Autodesk Inventor part; units mm, degrees
ref_plane "YZ Plane" through (0, 0, 0) normal (1, 0, 0) x (0, 1, 0)
ref_plane "XZ Plane" through (0, 0, 0) normal (0, 1, 0) x (-1, 0, 0)
ref_plane "XY Plane" through (0, 0, 0) normal (0, 0, 1) x (1, 0, 0)
sketch "Sketch1" plane through (0, 0, 0) normal (0, 1, 0) x (-1, 0, 0)
  line L0 (6.35, 0) -> (1365.25, 0)
  line L1 (1371.6, -6.35) -> (1371.6, -1365.25)
  line L2 (1365.25, -1371.6) -> (6.35, -1371.6)
  line L3 (0, -1365.25) -> (0, -6.35)
  line L4 (1346.2, -1346.2) -> (1346.2, -25.4)
  line L5 (1346.2, -25.4) -> (25.4, -25.4)
  line L6 (25.4, -25.4) -> (25.4, -1346.2)
  line L7 (25.4, -1346.2) -> (1346.2, -1346.2)
  line L8 (1320.8, -50.8) -> (1320.8, -1320.8)
  line L9 (1320.8, -1320.8) -> (50.8, -1320.8)
  line L10 (50.8, -1320.8) -> (50.8, -50.8)
  line L11 (50.8, -50.8) -> (1320.8, -50.8)
  line L12 (1320.8, -50.8) -> (1346.2, -25.4)
  line L13 (1320.8, -1320.8) -> (1346.2, -1346.2)
  line L14 (50.8, -1320.8) -> (25.4, -1346.2)
  line L15 (50.8, -50.8) -> (25.4, -25.4)
  line L16 (1219.2, -482.6) -> (1016, -482.6)
  line L17 (1016, -482.6) -> (1016, -889)
  line L18 (1016, -889) -> (1219.2, -889)
  line L19 (1219.2, -889) -> (1219.2, -482.6)
  line L20 (355.6, -482.6) -> (152.4, -482.6)
  line L21 (152.4, -482.6) -> (152.4, -889)
  line L22 (152.4, -889) -> (355.6, -889)
  line L23 (355.6, -889) -> (355.6, -482.6)
  line L24 (889, -1016) -> (482.6, -1016)
  line L25 (482.6, -1016) -> (482.6, -1219.2)
  line L26 (482.6, -1219.2) -> (889, -1219.2)
  line L27 (889, -1219.2) -> (889, -1016)
  line L28 (889, -152.4) -> (482.6, -152.4)
  line L29 (482.6, -152.4) -> (482.6, -355.6)
  line L30 (482.6, -355.6) -> (889, -355.6)
  line L31 (889, -355.6) -> (889, -152.4)
  circle A0 centre (685.8, -685.8) radius 254
  line L32 (889, -127) -> (482.6, -127)
  line L33 (457.2, -127) -> (457.2, -381)
  line L34 (457.2, -381) -> (914.4, -381)
  line L35 (914.4, -381) -> (914.4, -127)
  line L36 (1244.6, -457.2) -> (990.6, -457.2)
  line L37 (990.6, -457.2) -> (990.6, -914.4)
  line L38 (990.6, -914.4) -> (1244.6, -914.4)
  line L39 (1244.6, -889) -> (1244.6, -482.6)
  line L40 (914.4, -990.6) -> (457.2, -990.6)
  line L41 (457.2, -990.6) -> (457.2, -1244.6)
  line L42 (482.6, -1244.6) -> (889, -1244.6)
  line L43 (914.4, -1244.6) -> (914.4, -990.6)
  line L44 (381, -457.2) -> (127, -457.2)
  line L45 (127, -482.6) -> (127, -889)
  line L46 (127, -914.4) -> (381, -914.4)
  line L47 (381, -914.4) -> (381, -457.2)
  line L48 (152.4, -482.6) -> (50.8, -482.6)
  line L49 (127, -457.2) -> (50.8, -457.2)
  line L50 (152.4, -889) -> (50.8, -889)
  line L51 (127, -914.4) -> (50.8, -914.4)
  line L52 (355.6, -889) -> (381, -889)
  line L53 (355.6, -482.6) -> (381, -482.6)
  line L54 (457.2, -1244.6) -> (457.2, -1320.8)
  line L55 (482.6, -1219.2) -> (482.6, -1320.8)
  line L56 (889, -1219.2) -> (889, -1320.8)
  line L57 (914.4, -1244.6) -> (914.4, -1320.8)
  line L58 (1244.6, -914.4) -> (1320.8, -914.4)
  line L59 (1219.2, -889) -> (1320.8, -889)
  line L60 (1219.2, -482.6) -> (1320.8, -482.6)
  line L61 (1244.6, -457.2) -> (1320.8, -457.2)
  line L62 (889, -152.4) -> (889, -50.8)
  line L63 (914.4, -127) -> (914.4, -50.8)
  line L64 (482.6, -152.4) -> (482.6, -50.8)
  line L65 (457.2, -127) -> (457.2, -50.8)
  line L66 (889, -1016) -> (889, -990.6)
  line L67 (482.6, -1016) -> (482.6, -990.6)
  line L68 (1016, -889) -> (990.6, -889)
  line L69 (1016, -482.6) -> (990.6, -482.6)
  line L70 (889, -355.6) -> (889, -381)
  line L71 (482.6, -355.6) -> (482.6, -381)
  line L72 (914.4, -381) -> (990.6, -457.2)
  line L73 (990.6, -482.6) -> (889, -381)
  line L74 (990.6, -914.4) -> (914.4, -990.6)
  line L75 (889, -990.6) -> (990.6, -889)
  line L76 (381, -914.4) -> (457.2, -990.6)
  line L77 (482.6, -990.6) -> (381, -889)
  line L78 (457.2, -381) -> (381, -457.2)
  line L79 (482.6, -381) -> (381, -482.6)
  line L80 (1257.3, -50.8) -> (1320.8, -114.3)
  line L81 (1320.8, -1257.3) -> (1257.3, -1320.8)
  line L82 (50.8, -1257.3) -> (114.3, -1320.8)
  line L83 (50.8, -114.3) -> (114.3, -50.8)
  line L84 (68.7605, -132.2605) -> (132.2605, -68.7605)
  line L85 (68.7605, -1239.3395) -> (132.2605, -1302.8395)
  line L86 (1302.8395, -1239.3395) -> (1239.3395, -1302.8395)
  line L87 (1239.3395, -68.7605) -> (1302.8395, -132.2605)
  line L88 (1302.8395, -132.2605) -> (1320.8, -150.221)
  line L89 (1239.3395, -68.7605) -> (1221.379, -50.8)
  line L90 (1302.8395, -1239.3395) -> (1320.8, -1221.379)
  line L91 (1239.3395, -1302.8395) -> (1221.379, -1320.8)
  line L92 (132.2605, -1302.8395) -> (150.221, -1320.8)
  line L93 (68.7605, -1239.3395) -> (50.8, -1221.379)
  line L94 (132.2605, -68.7605) -> (150.221, -50.8)
  line L95 (68.7605, -132.2605) -> (50.8, -150.221)
  line L96 (1365.25, 0) -> (1371.6, -6.35)
  line L97 (1371.6, -1365.25) -> (1365.25, -1371.6)
  line L98 (6.35, -1371.6) -> (0, -1365.25)
  line L99 (6.35, 0) -> (0, -6.35)
  point P0 (0, 0)
  point P1 (1371.6, -1371.6)
  point P2 (1371.6, 0)
  point P3 (0, -1371.6)
  dimension "d0" = 1371.6
  dimension "d1" = 1371.6
  dimension "d2" = 25.4
  dimension "d3" = 25.4
  dimension "d4" = 203.2
  dimension "d5" = 406.4
  dimension "d6" = 203.2
  dimension "d7" = 406.4
  dimension "d8" = 406.4
  dimension "d9" = 203.2
  dimension "d10" = 406.4
  dimension "d11" = 203.2
  dimension "d12" = 101.6
  dimension "d13" = 101.6
  dimension "d14" = 101.6
  dimension "d15" = 101.6
  dimension "d16" = 431.8
  dimension "d17" = 431.8
  dimension "d18" = 431.8
  dimension "d19" = 431.8
  dimension "d20" = 508
  dimension "d21" = 25.4
  dimension "d22" = 25.4
  dimension "d23" = 25.4
  dimension "d24" = 25.4
  dimension "d25" = 45
  dimension "d26" = 63.5
  dimension "d27" = 45
  dimension "d28" = 45
  dimension "d29" = 45
  dimension "d30" = 25.4
  dimension "d31" = 25.4
  dimension "d32" = 25.4
  dimension "d33" = 25.4
  dimension "d34" = 6.35
  dimension "d35" = 6.35
  dimension "d36" = 6.35
  dimension "d37" = 6.35
  dimension "d38" = 6.35
  dimension "d39" = 6.35
  dimension "d40" = 6.35
  dimension "d41" = 6.35
extrude "Extrusion1" add sketch "Sketch1" along normal blind 5.08 contours L0 L96 L1 L97 L2 L98 L3 L99 | L13 L8 L12 L4 | L7 L14 L9 L13 | L12 L11 L15 L5 | L6 L15 L10 L14 | L9 L81 L8 | L8 L80 L11 | L10 L82 L9 | L81 L9 L91 L86 L90 L8 | L11 L83 L10 | L8 L88 L87 L89 L11 L80 | L82 L10 L93 L85 L92 L9 | L90 L86 L91 L9 L57 L43 L74 L38 L58 L8 | L83 L11 L94 L84 L95 L10 | L8 L61 L36 L72 L35 L63 L11 L89 L87 L88 | L92 L85 L93 L10 L51 L46 L76 L41 L54 L9 | L58 L38 L37 L68 L18 L59 L8 | L9 L56 L27 L66 L40 L43 L57 | L95 L84 L94 L11 L65 L33 L78 L44 L49 L10 | L8 L60 L16 L69 L37 L36 L61 | L63 L35 L34 L70 L31 L62 L11 | L54 L41 L40 L67 L25 L55 L9 | L10 L50 L22 L52 L47 L46 L51 | L59 L39 L60 L8 | L9 L55 L42 L56 | L49 L44 L47 L53 L20 L48 L10 | L11 L64 L29 L71 L34 L33 L65 | L62 L32 L64 L11 | L10 L48 L45 L50 | L74 L40 L75 L37 | L37 L73 L34 L72 | L76 L47 L77 L40 | L75 L40 L77 L47 L79 L34 L73 L37 | L78 L34 L79 L47
chamfer "Chamfer1" distance 1.524 angle 45 8 edges at (-1371.6, 5.08, -685.8) (-1371.6, 0, -685.8) (-685.8, 5.08, 0) (-685.8, 0, 0) (-685.8, 5.08, -1371.6) (-685.8, 0, -1371.6) (0, 5.08, -685.8) (0, 0, -685.8)
properties part number "Glass top X1" material "Glass"
Verification items for the finished model (mm, model axes). Round coordinates to 2 decimals unless told otherwise and drop trailing zeros. Order: outer loops, then holes, each group sorted by start corner. A loop starts at its lowest first (then second) coordinate and runs counter-clockwise, first axis right, second up. Notation, with made-up numbers: (1.5, -10.5) -> (44.5, -10.5) arc R21 cw to (44.5, 16.5) -> close; hole circle Ø5 at (-14.5, 59.25). An arc over 180 degrees is marked (long way). Put each result on its own line as item: value. Start each with the question number.
(1) Depth check by flat-ended pin: pin 1 Ø1 at (y, z) = (1, -867) entering from -X. Enter the tip coordinate at first touch or a pass-through.
(2) Material ranges on line 1 along Z through (x, y) = (-685.8, 2); line 2 along Z through (x, y) = (-685.8, 1.15); line 3 along X through (y, z) = (2.4, -1139), recorded low to high.
(3) Section check D-D (y = 2.45). Enter the section's corners in (x, z).
(4) Section check B-B (z = -685.8). Enter the section's corners in (x, y).
(5) Section check C-C (x = -685.8). Enter the section's corners in (y, z).
(6) Section check A-A (x = -1200). Enter the section's corners in (y, z).
Completed:
1. pin 1: stops at x = -1371.58
2. line 1: z = -1371.6 to -1244.6, -990.6 to -939.8, -431.8 to -381, -127 to 0
2. line 2: z = -1371.23 to -1244.6, -990.6 to -939.8, -431.8 to -381, -127 to -0.37
2. line 3: x = -1371.6 to -889, -482.6 to 0
3. outline: (-1371.6, -1365.25) -> (-1365.25, -1371.6) -> (-6.35, -1371.6) -> (0, -1365.25) -> (0, -6.35) -> (-6.35, 0) -> (-1365.25, 0) -> (-1371.6, -6.35) -> close; hole (-1244.6, -889) -> (-990.6, -889) -> (-990.6, -482.6) -> (-1244.6, -482.6) -> close; hole circle Ø508 at (-685.8, -685.8); hole (-889, -1244.6) -> (-482.6, -1244.6) -> (-482.6, -990.6) -> (-889, -990.6) -> close; hole (-889, -381) -> (-482.6, -381) -> (-482.6, -127) -> (-889, -127) -> close; hole (-381, -889) -> (-127, -889) -> (-127, -482.6) -> (-381, -482.6) -> close
4. outline: (-1371.6, 1.52) -> (-1370.08, 0) -> (-1244.6, 0) -> (-1244.6, 5.08) -> (-1370.08, 5.08) -> (-1371.6, 3.56) -> close; (-990.6, 0) -> (-939.8, 0) -> (-939.8, 5.08) -> (-990.6, 5.08) -> close; (-431.8, 0) -> (-381, 0) -> (-381, 5.08) -> (-431.8, 5.08) -> close; (-127, 0) -> (-1.52, 0) -> (0, 1.52) -> (0, 3.56) -> (-1.52, 5.08) -> (-127, 5.08) -> close
5. outline: (0, -1370.08) -> (1.52, -1371.6) -> (3.56, -1371.6) -> (5.08, -1370.08) -> (5.08, -1244.6) -> (0, -1244.6) -> close; (0, -990.6) -> (5.08, -990.6) -> (5.08, -939.8) -> (0, -939.8) -> close; (0, -431.8) -> (5.08, -431.8) -> (5.08, -381) -> (0, -381) -> close; (0, -127) -> (5.08, -127) -> (5.08, -1.52) -> (3.56, 0) -> (1.52, 0) -> (0, -1.52) -> close
6. outline: (0, -1370.08) -> (1.52, -1371.6) -> (3.56, -1371.6) -> (5.08, -1370.08) -> (5.08, -889) -> (0, -889) -> close; (0, -482.6) -> (5.08, -482.6) -> (5.08, -1.52) -> (3.56, 0) -> (1.52, 0) -> (0, -1.52) -> close
